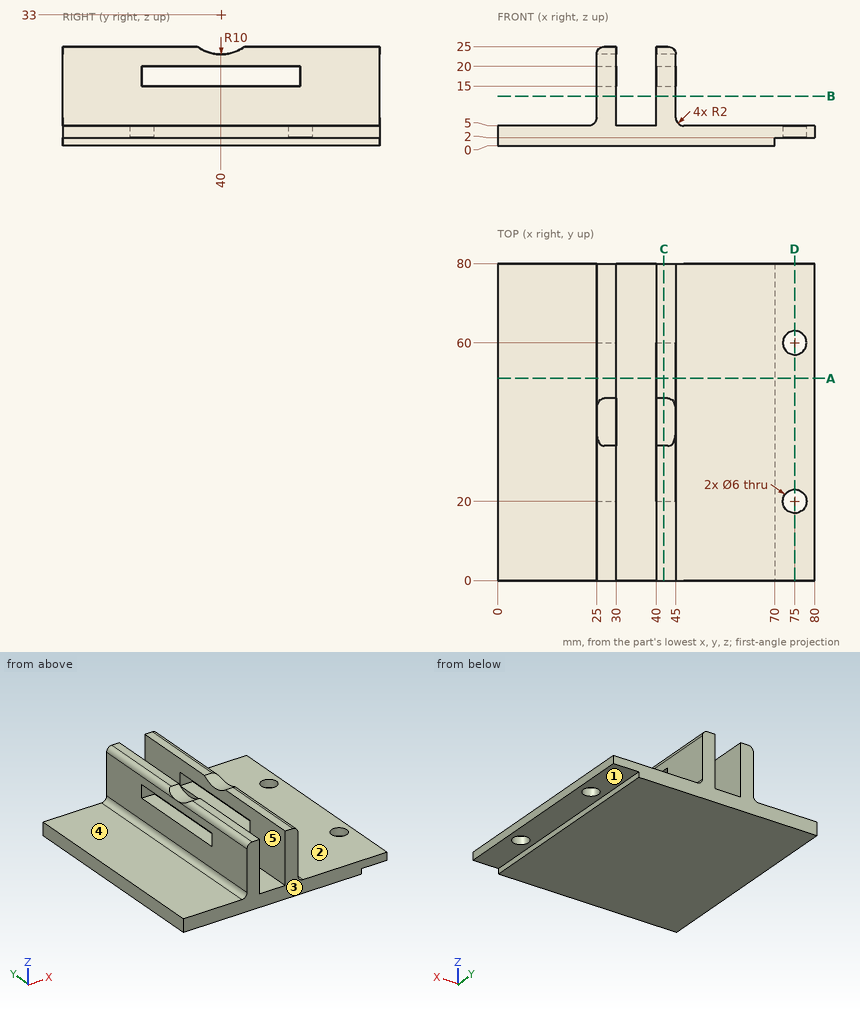
Drawing for the job (mm, zero at the part's lowest x, y, z). A direction names the side the tool comes from. Round coordinates to 2 decimals unless told otherwise and drop trailing zeros. Loops run counter-clockwise (first coordinate to the right, second up) from the corner with the lowest first, then second, coordinate; pieces in that order, holes last. Notation, with made-up numbers: (45, 45) -> (85, 45) arc R14 cw to (85, 71) -> close; hole circle Ø6 at (31, -3.75). An arc over 180 degrees is marked (long way). Use one line per item in the form item = value. Start each with the question number.
Item 1: Drill centre lines: line 1 along Y through (x, z) = (75, 3); line 2 along X through (y, z) = (9, 19.5); line 3 along Z through (x, y) = (28, 31.5). Where is each one in solid material? Low to high.
Item 2: Band-saw the part on D-D (x = 75). List the corners of the cut face in (y, z), plus the area to 3 significant figures.
Item 3: Band-saw the part on A-A (y = 51). List the corners of the cut face in (x, z).
Item 4: Band-saw the part on B-B (z = 12.5). List the corners of the cut face in (x, y), plus the area to 3 significant figures.
Item 5: Tool access for the marked faces 1, 2, 3, 4 and 5: list every direction of +Z, -Z, +X, -X, +Y, -Y with a clear straight run to the whole face (end or side of a thin tool).
Item 6: Drop flat-ended pins along their axis: pin 1 Ø3 at (y, z) = (41.5, 12.5) entering from +X; pin 2 Ø3 at (y, z) = (66.5, 19) entering from -X; pin 3 Ø8 at (x, y) = (76.5, 23.5) entering from -Z. Give the stop position or say it passes through.
Item 7: Band-saw the part on C-C (x = 42). List the corners of the cut face in (y, z).
Data:
q1.line_1 = 0 to 17, 23 to 57, 63 to 80
q1.line_2 = 25 to 30, 40 to 45
q1.line_3 = 0 to 15, 20 to 25
q2.outline = (0, 2) -> (17, 2) -> (17, 5) -> (0, 5) -> close; (23, 2) -> (57, 2) -> (57, 5) -> (23, 5) -> close; (63, 2) -> (80, 2) -> (80, 5) -> (63, 5) -> close
q2.area = 204 mm^2
q3.outline = (0, 0) -> (70, 0) -> (70, 2) -> (80, 2) -> (80, 5) -> (47, 5) arc R2 cw to (45, 7) -> (45, 15) -> (40, 15) -> (40, 5) -> (30, 5) -> (30, 15) -> (25, 15) -> (25, 7) arc R2 cw to (23, 5) -> (0, 5) -> close; (25, 20) -> (30, 20) -> (30, 25) -> (27, 25) arc R2 ccw to (25, 23) -> close; (40, 20) -> (45, 20) -> (45, 23) arc R2 ccw to (43, 25) -> (40, 25) -> close
q4.outline = (25, 0) -> (30, 0) -> (30, 80) -> (25, 80) -> close; (40, 0) -> (45, 0) -> (45, 80) -> (40, 80) -> close
q4.area = 800 mm^2
q5.face_1 = -Z, +X, +Y, -Y
q5.face_2 = +Z, +X, +Y, -Y
q5.face_3 = +Z, -Z, +X, -X, -Y
q5.face_4 = +Z, -X, +Y, -Y
q5.face_5 = +Z, +Y, -Y
q6.pin_1 = 45
q6.pin_2 = 25
q6.pin_3 = 2
q7.outline = (0, 0) -> (80, 0) -> (80, 25) -> (46, 25) arc R10 cw to (34, 25) -> (0, 25) -> close; hole (20, 15) -> (60, 15) -> (60, 20) -> (20, 20) -> close
